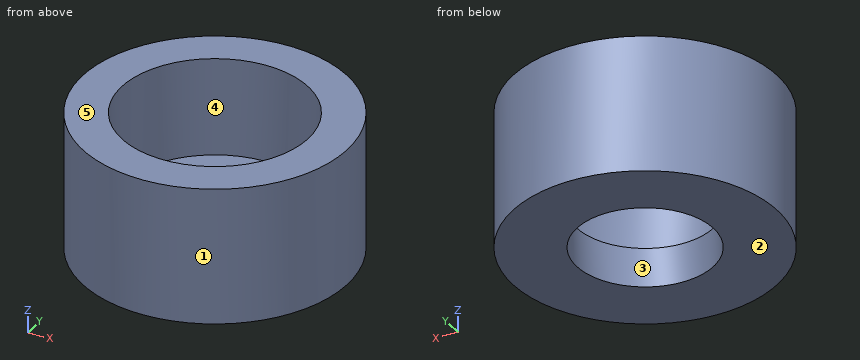
```python
from build123d import *

# Parameters (mm, degrees)
SKETCH1_R           = 8.598499948
SKETCH1_R_2         = 6.058499948
BOSS_EXTRUDE1_DEPTH = 6.35
SKETCH2_R           = 8.598499948
BOSS_EXTRUDE2_DEPTH = 2.54
SKETCH3_R           = 4.445
CUT_EXTRUDE1_DEPTH  = 9.89


with BuildPart() as part:
    # Sketch1 → Boss-Extrude1 (new body)
    with BuildSketch(Plane.XY):
        Circle(SKETCH1_R)
        Circle(SKETCH1_R_2, mode=Mode.SUBTRACT)
    extrude(amount=BOSS_EXTRUDE1_DEPTH)

    # Sketch2 → Boss-Extrude2 (add)
    with BuildSketch(Plane.XY):
        Circle(SKETCH2_R)
    extrude(amount=-BOSS_EXTRUDE2_DEPTH)

    # Sketch3 → Cut-Extrude1 (cut, through all)
    with BuildSketch(Plane(origin=(0, 0, -2.54), x_dir=(-1, 0, 0), z_dir=(0, 0, -1))):
        Circle(SKETCH3_R)
    extrude(amount=-CUT_EXTRUDE1_DEPTH, mode=Mode.SUBTRACT)


solid = part.part
```
Geometry check sheet. Reference: the model listing, model coordinates, mm. Face numbers are marked on the shaded views. A direction names the side the tool comes from. Coordinates: 2 decimals unless noted, no trailing zeros. Write each loop counter-clockwise with the first axis right and the second up, starting at its lowest first coordinate (ties: lowest second). Pieces come first, ordered by that corner, then holes. Notation, with made-up numbers: (30, 41) -> (73, 41) arc R19 ccw to (73, 69) -> close; hole circle Ø3 at (42.25, 87). An arc over 180 degrees is marked (long way). Use CSV: the item, a comma, the result in double quotes. Start each with the question number.
Item 1: Depth check by flat-ended pin: pin 1 Ø7 at (x, y) = (0, 0) entering from -Z; pin 2 Ø6 at (x, y) = (1, -2.5) entering from +Z; pin 3 Ø1 at (y, z) = (-5.5, 1) entering from +X; pin 4 Ø1 at (y, z) = (-5.5, 4.5) entering from -X. Enter the tip coordinate at first touch or a pass-through.
Item 2: Cross-section at D-D, the plane y = -5.5. Record the cut outline in (x, z).
Item 3: Mould release check, pull along Y, two halves, no side actions. Record for the marked faces 1, 2 and 3: released by +Y, released by -Y, zero draft, split by the parting line, or undercut.
Item 4: Cross-section at C-C, the plane z = 1. Record the cut outline in (x, y), plus the area to 3 significant figures.
Item 5: Thickness scan on line 1 (Y direction, x = 0, z = 2.5); line 2 (Z direction, x = -5, y = 2); line 3 (X direction, y = -3.75, z = 5). Record the ranges inside material, lowest first.
Item 6: Set-up check for the marked faces 4 and 5: record each of +Z, -Z, +X, -X, +Y, -Y from which the full face is reachable in a straight line by a thin tool's end or side.
Answers:
1,pin 1,"through"
1,pin 2,"z = 0"
1,pin 3,"x = 7"
1,pin 4,"x = -7"
2,outline,"(-6.61, -2.54) -> (6.61, -2.54) -> (6.61, 6.35) -> (2.54, 6.35) -> (2.54, 0) -> (-2.54, 0) -> (-2.54, 6.35) -> (-6.61, 6.35) -> close"
3,face 1,"split by the parting line"
3,face 2,"zero draft"
3,face 3,"undercut"
4,outline,"circle Ø17.2 at (0, 0); hole circle Ø12.12 at (0, 0)"
4,area,"117 mm^2"
5,line 1,"-8.6 to -6.06, 6.06 to 8.6"
5,line 2,"-2.54 to 0"
5,line 3,"-7.74 to -4.76, 4.76 to 7.74"
6,face 4,"+Z"
6,face 5,"+Z, +X, -X, +Y, -Y"
